```python
from build123d import *

# Parameters (mm, degrees)
F0_W     = 42.3
F0_H     = 42.3
F1_DEPTH = 34
F2_R     = 11
F3_DEPTH = 2
F4_R     = 2.5
F5_DEPTH = 14
F6_SIZE  = 5.65
F7_R     = 1.75
F8_DEPTH = 4.5


with BuildPart() as f1:
    # F0 (on Top) → F1 (new body)
    with BuildSketch(Plane.XY):
        Rectangle(F0_W, F0_H)
    extrude(amount=F1_DEPTH)

    # F2 (on face) → F3 (join)
    with BuildSketch(Plane.XY.offset(34)):
        Circle(F2_R)
    extrude(amount=F3_DEPTH)

    # F4 (on face) → F5 (join)
    with BuildSketch(Plane.XY.offset(36)):
        Circle(F4_R)
    extrude(amount=F5_DEPTH)

    # F6
    f6_edges = [f1.edges().sort_by_distance(p)[0] for p in [
        (21.15, 21.15, 17),
        (-21.15, 21.15, 17),
        (21.15, -21.15, 17),
        (-21.15, -21.15, 17),
    ]]
    chamfer(f6_edges, length=F6_SIZE)

    # F7 (on face) → F8 (cut)
    with BuildSketch(Plane.XY.offset(34)):
        with Locations((16, 15.5)):
            Circle(F7_R)
        with Locations((-16, 15.5)):
            Circle(F7_R)
        with Locations((16, -15.5)):
            Circle(F7_R)
        with Locations((-16, -15.5)):
            Circle(F7_R)
    extrude(amount=-F8_DEPTH, mode=Mode.SUBTRACT)


solid = f1.part
```
Geometry: final body of the model. Coordinates: model frame, mm. A direction names the side the tool comes from. Coordinates: 2 decimals unless noted, no trailing zeros. Write each loop counter-clockwise with the first axis right and the second up, starting at its lowest first coordinate (ties: lowest second). Pieces come first, ordered by that corner, then holes. Notation, with made-up numbers: M -10.5,69 L 39.5,69 A13 cw 39.5,73 Z; hole C 37,86.25 d8. An arc over 180 degrees is marked long. Use CSV: the item, a comma, the result in double quotes. Start each with the question number.
1. Cut plane A-A on z = 23. Return the cut outline in (x, y), plus the area to 3 significant figures.
2. Cut plane B-B on y = 0. Return the cut outline in (x, z).
3. Reachability of faces 1 (the face through (21.15, 0, 17)), 2 (the face through (-16.228, 17.235, 31.782)) from +Z, -Z, +X, -X, +Y, -Y: full face, straight path, thin tool, end or side. Return the list, or none.
4. Mould query, pull axis Y, two halves, no side actions, for faces 3 (the face through (-18.29, -18.36, 16.76)), 4 (the face through (15.772, -13.765, 31.782)), 5 (the face through (16, -15, 29.5)), 6 (the face through (-18.29, 18.36, 16.76)). Classes: pulls with the +Y half, pulls with the -Y half, needs draft (parallel to the pull), parting line crosses it, or undercut.
5. Cut plane D-D on x = -5.5. Return the cut outline in (y, z).
6. Ray query, probe 1 along Y at (x, z) = (16, 30); probe 2 along X at (y, z) = (-15, 33); probe 3 along Y at (x, z) = (17.5, 31). Return the intervals inside material, ascending.
7. First-contact query: P1, Ø5, axis at x = -6, y = 1.5, coming from the +Z side; P2, Ø1, axis at x = 13, y = -11.5, coming from the +Z side; P3, Ø1, axis at x = -16.5, y = -15, coming from the +Z side. Flat tips, straight axial feed; report the tip coordinate or a pass-through.
Entries:
1,outline,"M -21.15,-15.5 L -15.5,-21.15 L 15.5,-21.15 L 21.15,-15.5 L 21.15,15.5 L 15.5,21.15 L -15.5,21.15 L -21.15,15.5 Z"
1,area,"1,730 mm²"
2,outline,"M -21.15,0 L 21.15,0 L 21.15,34 L 11,34 L 11,36 L 2.5,36 L 2.5,50 L -2.5,50 L -2.5,36 L -11,36 L -11,34 L -21.15,34 Z"
3,face 1,"+Z, -Z, +X, +Y, -Y"
3,face 2,"+Z"
4,face 3,"pulls with the -Y half"
4,face 4,"undercut"
4,face 5,"undercut"
4,face 6,"pulls with the +Y half"
5,outline,"M -21.15,0 L 21.15,0 L 21.15,34 L 9.53,34 L 9.53,36 L -9.53,36 L -9.53,34 L -21.15,34 Z"
6,probe 1,"-20.65 to -17.25, -13.75 to 13.75, 17.25 to 20.65"
6,probe 2,"-21.15 to -17.68, -14.32 to 14.32, 17.68 to 21.15"
6,probe 3,"-19.15 to -16.4, -14.6 to 14.6, 16.4 to 19.15"
7,P1,"z = 36"
7,P2,"z = 34"
7,P3,"z = 29.5"
